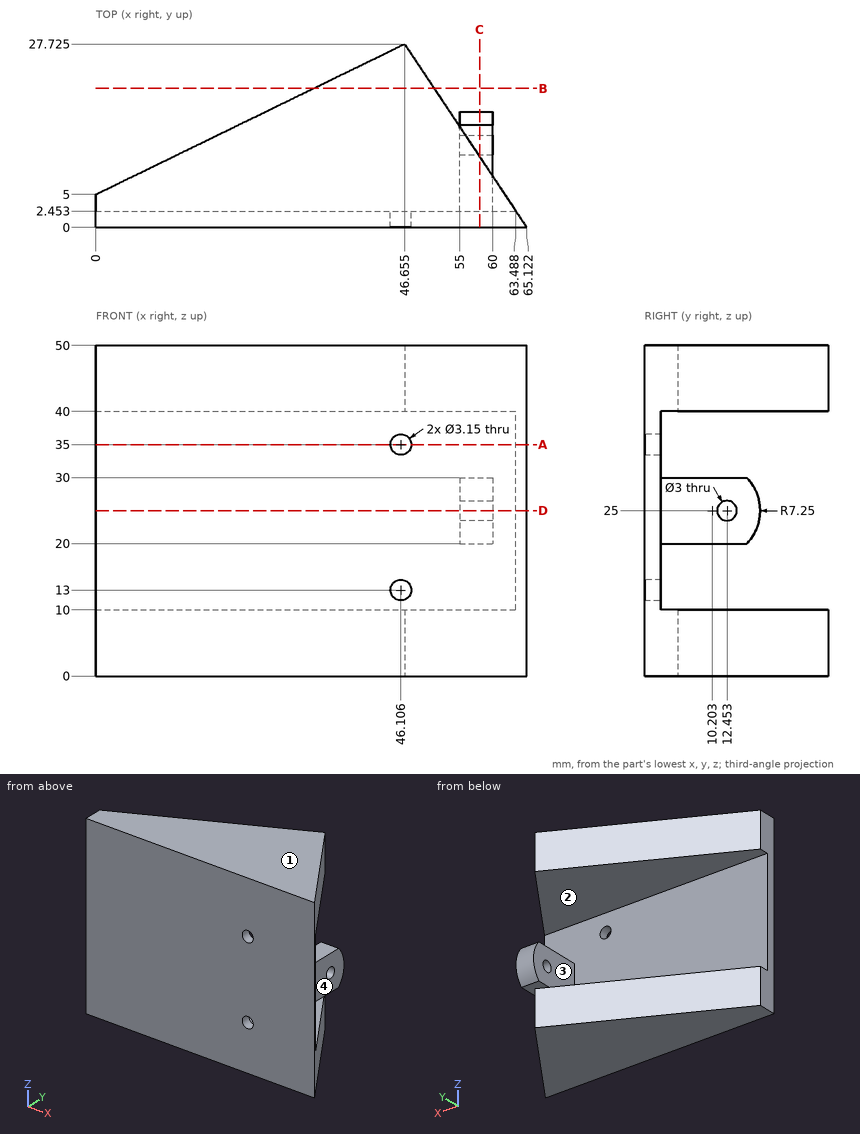
Here's the drawing with two shaded views (mm, measured from the low corner). I have some questions. A direction names the side the tool comes from. Give positions to 0.01 mm unless a question says otherwise; leave off trailing zeros. Write each loop counter-clockwise with the first axis right and the second up, starting at its lowest first coordinate (ties: lowest second). Pieces come first, ordered by that corner, then holes. Notation, with made-up numbers: (49, 81.5) -> (86, 81.5) arc R20 ccw to (86, 101.5) -> close; hole circle Ø4 at (20, 19.5). An arc over 180 degrees is marked (long way). Use one line per item in the form item = value. Start each with the question number.
1. Imagine slicing it at D-D on z = 25. List the corners of the cut face in (x, y) for me.
2. If I drill on L1, parallel to Z at x = 46.5, y = 22.75; L2, parallel to Y at x = 58, z = 25; L3, parallel to Y at x = 42, z = 17.5, over which ranges is the centre line in solid material (lowest first)?
3. On a 3-axis mill with a long thin cutter (end or side, diameter ignored), from which of +Z, -Z, +X, -X, +Y, -Y can I reach the whole of each face in a straight line? I mean the marked faces 1, 2, 3 and 4. Say none if no direction works.
4. Imagine slicing it at C-C on x = 58. List the corners of the cut face in (y, z) for me, plus the area to 3 significant figures.
5. Imagine slicing it at B-B on y = 21. List the corners of the cut face in (x, z) for me, plus the area to 3 significant figures.
6. Will these pins go through, and if not, where does the flat tip stop? pin 1 Ø3 at (y, z) = (11.5, 24) entering from +X; pin 2 Ø3 at (y, z) = (8.5, 24) entering from -X.
7. Imagine slicing it at A-A on z = 35. List the corners of the cut face in (x, y) for me.
Entries:
q1.outline = (0, 0) -> (65.12, 0) -> (63.49, 2.45) -> (60, 2.45) -> (60, 10.95) -> (55, 10.95) -> (55, 2.45) -> (0, 2.45) -> close; (55, 13.95) -> (60, 13.95) -> (60, 17.45) -> (55, 17.45) -> close
q2.L1 = 0 to 10, 40 to 50
q2.L2 = 0 to 10.95, 13.95 to 17.45
q2.L3 = 0 to 2.45
q3.face_1 = +Z, +X, -X, +Y, -Y
q3.face_2 = +X, -X, +Y
q3.face_3 = -X, +Y
q3.face_4 = +X, +Y
q4.outline = (0, 0) -> (10.69, 0) -> (10.69, 10) -> (2.45, 10) -> (2.45, 20) -> (15.45, 20) arc R7.25 ccw to (15.45, 30) -> (2.45, 30) -> (2.45, 40) -> (10.69, 40) -> (10.69, 50) -> (0, 50) -> close; hole circle Ø3 at (12.45, 25)
q4.area = 424 mm²
q5.outline = (32.85, 0) -> (51.13, 0) -> (51.13, 10) -> (32.85, 10) -> close; (32.85, 40) -> (51.13, 40) -> (51.13, 50) -> (32.85, 50) -> close
q5.area = 366 mm²
q6.pin_1 = 60
q6.pin_2 = 55
q7.outline = (0, 0) -> (44.53, 0) -> (44.53, 2.45) -> (0, 2.45) -> close; (47.68, 0) -> (65.12, 0) -> (63.49, 2.45) -> (47.68, 2.45) -> close
